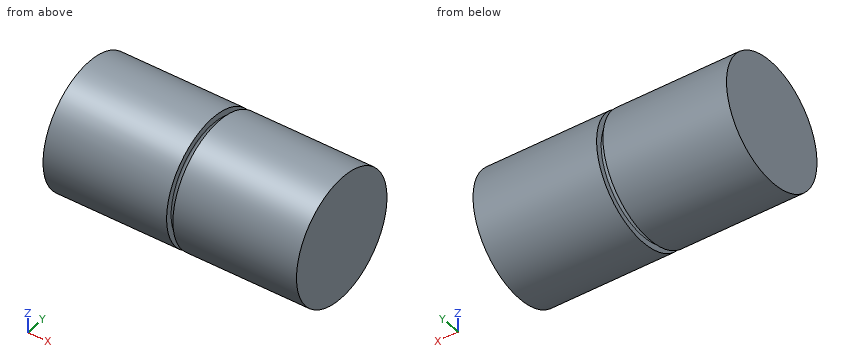
Autodesk Fusion 360 part; units mm, degrees
sketch "Sketch1" plane through (0, 0, 0) normal (0, 0, 1) x (1, 0, 0)
  line L0 (100, 0) -> (100, 50)
  line L1 (100, 50) -> (2.5, 50)
  line L2 (2.5, 50) -> (2.5, 45)
  arc A0 (0, 42.5) -> (2.5, 45) centre (0, 45) ccw
  line L3 (0, 0) -> (100, 0) construction
  line L4 (0, 0) -> (0, 45) construction
  line L5 (0, 42.5) -> (100, 42.5) construction
  line L6 (100, 0) -> (100, -50) construction
  line L7 (100, -50) -> (2.5, -50) construction
  line L8 (2.5, -50) -> (2.5, -45) construction
  arc A1 (2.5, -45) -> (0, -42.5) centre (0, -45) ccw construction
  arc A2 (-2.5, 45) -> (0, 42.5) centre (0, 45) ccw
  line L9 (-2.5, 50) -> (-2.5, 45)
  line L10 (-100, 50) -> (-2.5, 50)
  line L11 (-100, 0) -> (-100, 50)
  line L12 (-100, 0) -> (-100, -50) construction
  line L13 (-100, -50) -> (-2.5, -50) construction
  line L14 (-2.5, -50) -> (-2.5, -45) construction
  arc A3 (0, -42.5) -> (-2.5, -45) centre (0, -45) ccw construction
  line L15 (100, 0) -> (-100, 0)
  dimension "Notch_Radius" = 2.5
  dimension "Notch_Height" = 7.5
  dimension "Bar_Diameter" = 100
  dimension "Bar_Length" = 200
revolve "Revolve1" add sketch "Sketch1" angle 360 about axis through (0, 0, 0) along (1, 0, 0)
The listing builds one solid part. Answer for the finished solid, in the listing's coordinates (mm). Round coordinates to 2 decimals unless told otherwise and drop trailing zeros. Order: outer loops, then holes, each group sorted by start corner. A loop starts at its lowest first (then second) coordinate and runs counter-clockwise, first axis right, second up. Notation, with made-up numbers: (66.25, -22.5) -> (70.25, -22.5) arc R7 ccw to (70.25, -16.5) -> close; hole circle Ø3 at (-21.75, 82.25). An arc over 180 degrees is marked (long way). Put each result on its own line as item: value.
Q1. Each of these flat-tipped pins is pushed along its axis until it touches: P1, Ø3, axis at x = -40, z = 17, coming from the +Y side; P2, Ø5, axis at x = 52, y = 39.5, coming from the +Z side; P3, Ø3, axis at x = -39.5, y = 9, coming from the -Z side. Where does it stop, or does it pass through?
Results list:
P1: y = 47.54
P2: z = 33.63
P3: z = -49.43
Q2. Section A-A, the plane x = 55 is taken. Write down the section's boundary in (y, z), and give its area (3 significant figures).
Results list:
outline: circle Ø100 at (0, 0)
area: 7,850 mm^2
Q3. Consider line 1 along X through (y, z) = (-26, -38); line 2 along X through (y, z) = (-35.5, -25); line 3 along Y through (x, z) = (-61, -2). Determine where each line is inside the solid, lowest interval first.
Results list:
line 1: -100 to -2.5, 2.5 to 100
line 2: -100 to -1.94, 1.94 to 100
line 3: -49.96 to 49.96
